```python
from build123d import *

# Parameters (mm, degrees)
F0_W     = 1800
F0_H     = 800
F1_DEPTH = 25
F2_W     = 60
F2_H     = 60
F3_DEPTH = 800
F4_W     = 80
F4_H     = 600
F5_DEPTH = 25
F6_SIZE  = 20


with BuildPart() as f1:
    # F0 (on Top) → F1 (new body)
    with BuildSketch(Plane.XY):
        with Locations((900, -400)):
            Rectangle(F0_W, F0_H)
    extrude(amount=F1_DEPTH)

    # F2 (on face) → F3 (join)
    with BuildSketch(Plane(origin=(0, 0, 0), x_dir=(1, 0, 0), z_dir=(0, 0, -1))):
        with Locations((60, 550)):
            Rectangle(F2_W, F2_H)
        with Locations((1740, 550)):
            Rectangle(F2_W, F2_H)
    extrude(amount=F3_DEPTH)

    # F4 (on face) → F5 (join)
    with BuildSketch(Plane(origin=(0, 0, -800), x_dir=(1, 0, 0), z_dir=(0, 0, -1))):
        with Locations((60, 390)):
            Rectangle(F4_W, F4_H)
        with Locations((1740, 390)):
            Rectangle(F4_W, F4_H)
    extrude(amount=F5_DEPTH)

    # F6
    f6_edges = [f1.edges().sort_by_distance(p)[0] for p in [
        (1740, -90, -800),
        (60, -90, -800),
        (60, -690, -800),
        (1740, -690, -800),
    ]]
    chamfer(f6_edges, length=F6_SIZE)


solid = f1.part
```
For this review, take the finished solid that the model builds, in its own axes (mm). A direction names the side the tool comes from. Give positions to 0.01 mm unless a question says otherwise; leave off trailing zeros. Write each loop counter-clockwise with the first axis right and the second up, starting at its lowest first coordinate (ties: lowest second). Pieces come first, ordered by that corner, then holes. Notation, with made-up numbers: M -39,6 L 7,6 A25 ccw 7,40 Z; hole C 8,3.25 d2. An arc over 180 degrees is marked long. Answer as a JSON object with one key per item and string values. Group by question number.
Item 1: Consider section C-C on x = 518.5. Write out the cut boundary in (y, z), plus the area to 3 significant figures.
Item 2: Tool access review of faces 4 (the flat face through (60, -580, -394)), 5 (the flat face through (90, -550, -394)), 6 (the flat face through (60, -520, -394)): name each direction out of +Z, -Z, +X, -X, +Y, -Y from which nothing blocks a thin tool from reaching the whole face with its end or side.
Item 3: Consider section B-B on z = -95. Write out the cut boundary in (x, y).
Item 4: For probe 1 along Z at (x, y) = (1719, -350.5); probe 2 along X at (y, z) = (-567, -333); probe 3 along Z at (x, y) = (1249, -473), list the stretches that pass through material, from the lowest coordinate up. Write a range as [from, to].
Item 5: For pin 1 Ø12.5 at (y, z) = (-481, -816) entering from -X; pin 2 Ø1 at (x, y) = (1408.5, -459) entering from -Z; pin 3 Ø4 at (x, z) = (1747.5, -823.5) entering from -Y, all flat-tipped, find the tip position at first contact; note any pin that passes through.
Item 6: Consider section A-A on y = -457. Write out the cut boundary in (x, z).
Item 7: Draft analysis for pull direction Z (two halves, no side actions). For faces 1 (the flat face through (887, -394, 25)), 2 (the flat face through (30, -550, -394)), 3 (the flat face through (59, -394, -825)), state which applies: +Z half, -Z half, draft (parallel to the pull), parting line (faces both ways), or undercut.
Check result:
{
 "1": {"outline": "M -800,0 L 0,0 L 0,25 L -800,25 Z", "area": "20,000 mm^2"},
 "2": {"face 4": "+X, -X, -Y", "face 5": "+Y, -Y", "face 6": "+X, -X, +Y"},
 "3": {"outline": "M 30,-580 L 90,-580 L 90,-520 L 30,-520 Z; M 1710,-580 L 1770,-580 L 1770,-520 L 1710,-520 Z"},
 "4": {"probe 1": "z = [-825, -800], [0, 25]", "probe 2": "x = [30, 90], [1710, 1770]", "probe 3": "z = [0, 25]"},
 "5": {"pin 1": "stops at x = 20", "pin 2": "stops at z = 0", "pin 3": "stops at y = -690"},
 "6": {"outline": "M 0,0 L 1800,0 L 1800,25 L 0,25 Z; M 20,-825 L 100,-825 L 100,-800 L 20,-800 Z; M 1700,-825 L 1780,-825 L 1780,-800 L 1700,-800 Z"},
 "7": {"face 1": "+Z half", "face 2": "undercut", "face 3": "-Z half"}
}
